from build123d import *

# Parameters (mm, degrees)
BASETUBER_DEPTH    = 76.2
CUT_EXTRUDE1_REACH = 78.2
SKETCH2_R          = 9.525


with BuildPart() as part:
    # Sketch1 → BaseTubeR (new body, symmetric)
    with BuildSketch(Plane.XY):
        with BuildLine():
            Line((19.05, 0), (57.15, 0))
            ThreePointArc((57.15, 0), (70.620384182, 5.579615818), (76.2, 19.05))
            Line((76.2, 19.05), (76.2, 107.95))
            ThreePointArc((76.2, 107.95), (70.620384182, 121.420384182), (57.15, 127))
            Line((57.15, 127), (19.05, 127))
            ThreePointArc((19.05, 127), (5.579615818, 121.420384182), (0, 107.95))
            Line((0, 107.95), (0, 19.05))
            ThreePointArc((0, 19.05), (5.579615818, 5.579615818), (19.05, 0))
        make_face()
        with BuildLine():
            Line((19.05, 9.525), (57.15, 9.525))
            ThreePointArc((57.15, 9.525), (63.885192091, 12.314807909), (66.675, 19.05))
            Line((66.675, 19.05), (66.675, 107.95))
            ThreePointArc((66.675, 107.95), (63.885192091, 114.685192091), (57.15, 117.475))
            Line((57.15, 117.475), (19.05, 117.475))
            ThreePointArc((19.05, 117.475), (12.314807909, 114.685192091), (9.525, 107.95))
            Line((9.525, 107.95), (9.525, 19.05))
            ThreePointArc((9.525, 19.05), (12.314807909, 12.314807909), (19.05, 9.525))
        make_face(mode=Mode.SUBTRACT)
    extrude(amount=BASETUBER_DEPTH, both=True)

    # Sketch2 → Cut-Extrude1 (cut, up to next)
    with BuildSketch(Plane.ZY, mode=Mode.PRIVATE) as cut_extrude1_sk1:
        with Locations((-38.1, 31.75)):
            Circle(SKETCH2_R)
    cut_extrude1_tool1 = extrude(cut_extrude1_sk1.sketch, amount=-CUT_EXTRUDE1_REACH, mode=Mode.PRIVATE) & part.part
    add(cut_extrude1_tool1.solids().sort_by_distance((0, 31.75, -38.1))[0], mode=Mode.SUBTRACT)


solid = part.part
Part model, mm, in its own coordinate system. A direction names the side the tool comes from. Give positions to 0.01 mm unless a question says otherwise; leave off trailing zeros. Write each loop counter-clockwise with the first axis right and the second up, starting at its lowest first coordinate (ties: lowest second). Pieces come first, ordered by that corner, then holes.
1) Cut at A-A on y = 87. Write the cut outline in (x, z) (3 decimals), then the cut area to 3 significant figures.
Resolved:
outline: (0, -76.2) - (9.525, -76.2) - (9.525, 76.2) - (0, 76.2) - close; (66.675, -76.2) - (76.2, -76.2) - (76.2, 76.2) - (66.675, 76.2) - close
area: 2,900 mm2
2) Pin check, flat tips, straight feed: pin 1 (4 mm diameter, centred on x = 67, z = -22, fed in from -Y); pin 2 (12 mm diameter, centred on x = 65.5, z = 19, fed in from -Y); pin 3 (4 mm diameter, centred on x = 62, z = -10, fed in from -Y). Stop position of each tip, or through.
Resolved:
pin 1: stops at y = 1.69
pin 2: stops at y = 0.15
pin 3: stops at y = 0.21
3) Cut at D-D on y = 31.75. Write the cut outline in (x, z) (3 decimals), then the cut area to 3 significant figures.
Resolved:
outline: (0, -76.2) - (9.525, -76.2) - (9.525, -47.625) - (0, -47.625) - close; (0, -28.575) - (9.525, -28.575) - (9.525, 76.2) - (0, 76.2) - close; (66.675, -76.2) - (76.2, -76.2) - (76.2, 76.2) - (66.675, 76.2) - close
area: 2,720 mm2
4) Probe L1, parallel to X at y = 21.5, z = -19 (3 decimals); L2, parallel to Y at x = 32, z = -33.5 (3 decimals); L3, parallel to Z at x = 6, y = 31. List the from-to ranges inside material, lowest first.
Resolved:
L1: x = 0 to 9.525, 66.675 to 76.2
L2: y = 0 to 9.525, 117.475 to 127
L3: z = -76.2 to -47.6, -28.6 to 76.2
5) Cut at C-C on x = 43.5. Write the cut outline in (y, z) (3 decimals).
Resolved:
outline: (0, -76.2) - (9.525, -76.2) - (9.525, 76.2) - (0, 76.2) - close; (117.475, -76.2) - (127, -76.2) - (127, 76.2) - (117.475, 76.2) - close
6) Cut at B-B on z = -7.5. Write the cut outline in (x, y) (3 decimals), then the cut area to 3 significant figures.
Resolved:
outline: (0, 19.05) arc R19.05 ccw to (19.05, 0) - (57.15, 0) arc R19.05 ccw to (76.2, 19.05) - (76.2, 107.95) arc R19.05 ccw to (57.15, 127) - (19.05, 127) arc R19.05 ccw to (0, 107.95) - close; hole (9.525, 19.05) arc R9.525 ccw to (19.05, 9.525) - (57.15, 9.525) arc R9.525 ccw to (66.675, 19.05) - (66.675, 107.95) arc R9.525 ccw to (57.15, 117.475) - (19.05, 117.475) arc R9.525 ccw to (9.525, 107.95) - close
area: 3,270 mm2
7) Which spindle directions (+Z, -Z, +X, -X, +Y, -Y) get a long thin tool onto all of the face, cutting with end or side? Do faces 5 (the face through (63.81, 12.24, 1.07)), 6 (the face through (4.7, 23.3, -33.7)), 7 (the face through (5.73, 121.57, 1.07)). Say none if no direction does.
Resolved:
face 5: +Z, -Z
face 6: -X
face 7: +Z, -Z, -X, +Y
8) Two-plate mould, pull along X, no slides. Class faces 1 (the face through (0, 64, 1)), 2 (the face through (70.77, 121.27, 1.07)), 3 (the face through (38, 117.475, 1)), 4 (the face through (12.24, 12.39, 1.07)): released by +X, released by -X, zero draft, split by the parting line, or undercut.
Resolved:
face 1: released by -X
face 2: released by +X
face 3: undercut
face 4: undercut
